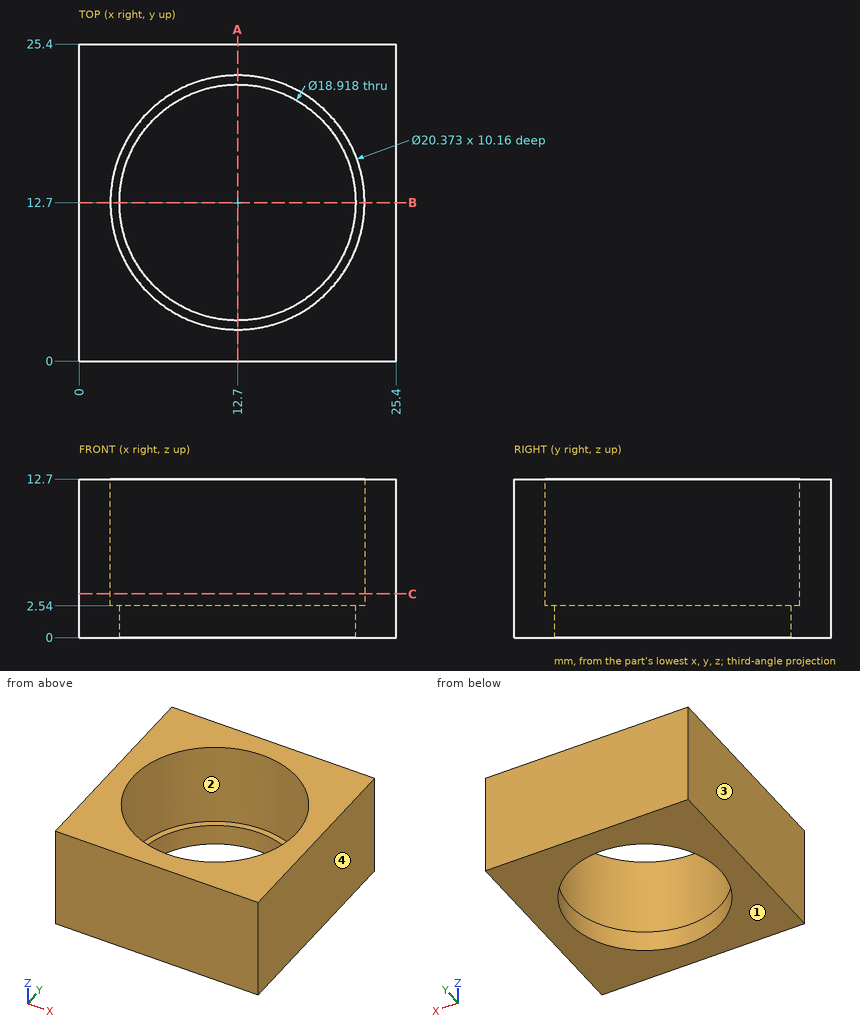
Here's the drawing with two shaded views (mm, measured from the low corner). I have some questions. Coordinates: 2 decimals unless noted, no trailing zeros. Write each loop counter-clockwise with the first axis right and the second up, starting at its lowest first coordinate (ties: lowest second). Pieces come first, ordered by that corner, then holes.
Item 1: I want a section at C-C on z = 3.5. Write out the boundary of the cut face in (x, y), and give its area (3 significant figures).
Item 2: If we mould it in two halves opening along X, with no side actions, what happens to the marked faces 1, 2, 3 and 4? For each: +X half, -X half, draft (parallel to the pull), parting line (faces both ways), or undercut.
Item 3: If I drill on line 1 (Y direction, x = 12.7, z = 2); line 2 (Y direction, x = 20.5, z = 6.25); line 3 (X direction, y = 15.25, z = 6.75), over which ranges is the centre line in solid material (lowest first)?
Item 4: I want a section at A-A on x = 12.7. Write out the boundary of the cut face in (y, z).
Findings below:
1. outline: (0, 0) - (25.4, 0) - (25.4, 25.4) - (0, 25.4) - close; hole circle Ø20.37 at (12.7, 12.7)
1. area: 319 mm2
2. face 1: draft
2. face 2: undercut
2. face 3: -X half
2. face 4: +X half
3. line 1: y = 0 to 3.24, 22.16 to 25.4
3. line 2: y = 0 to 6.15, 19.25 to 25.4
3. line 3: x = 0 to 2.84, 22.56 to 25.4
4. outline: (0, 0) - (3.24, 0) - (3.24, 2.54) - (2.51, 2.54) - (2.51, 12.7) - (0, 12.7) - close; (22.16, 0) - (25.4, 0) - (25.4, 12.7) - (22.89, 12.7) - (22.89, 2.54) - (22.16, 2.54) - close
